Work out the finished part from the listing and answer in its coordinate system (mm). Face numbers are marked on the shaded views. A direction names the side the tool comes from. Coordinates: 2 decimals unless noted, no trailing zeros. Order: outer loops, then holes, each group sorted by start corner. A loop starts at its lowest first (then second) coordinate and runs counter-clockwise, first axis right, second up. Notation, with made-up numbers: (64.5, 21.5) - (70.5, 21.5) arc R28 ccw to (70.5, 58.5) - close; hole circle Ø4 at (50, -33). An arc over 180 degrees is marked (long way). Answer as a JSON object with one key per item and string values. Group by question number.
1) The mould has two halves that part along X. Classify the marked faces 1, 2 and 3: released by +X, released by -X, zero draft, split by the parting line, or undercut.
2) Each of these flat-tipped pins is pushed along its axis until it touches: P1, Ø10, axis at x = 10, y = 6.5, coming from the +Z side (3 decimals); P2, Ø3.5, axis at y = 19.05, z = 79.248, coming from the +X side; P3, Ø4, axis at x = -9, y = 8.5, coming from the -Z side; P4, Ø4.5, axis at y = 17.74, z = 10.92, coming from the -X side. Where does it stop, or does it pass through?
3) Section D-D (z = 9.5) is taken. Give the vertices of the cut face in (x, y).
4) Section C-C (x = -27.5) is taken. Give the vertices of the cut face in (y, z) (3 decimals), plus the area to 3 significant figures.
5) A tool of negligible diameter and unlimited length cuts with its end or side. For the marked faces 4 and 5, from which of +Z, -Z, +X, -X, +Y, -Y can it reach the whole face along a straight path? Write none if from no direction.
6) Section B-B (y = 23) is taken. Give the vertices of the cut face in (x, z) (3 decimals).
7) Find the intervals of material crossed by line 1 along X through (y, z) = (9.5, 63); line 2 along Y through (x, z) = (22.5, 16); line 3 along Y through (x, z) = (35.8, 52.07), in increasing order.
8) Section A-A (z = 52.07) is taken. Give the vertices of the cut face in (x, y), plus the area to 3 significant figures.
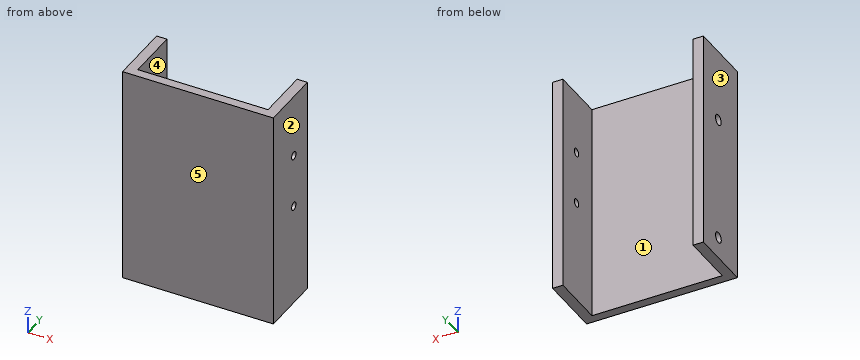
from build123d import *

# Parameters (mm, degrees)
BOSS_EXTRUDE3_DEPTH = 111.125
SKETCH4_R           = 2.667
CUT_EXTRUDE1_DEPTH  = 136.634929771
SKETCH5_R           = 2.667
CUT_EXTRUDE2_DEPTH  = 136.634929771
SKETCH6_R           = 2.032
CUT_EXTRUDE3_DEPTH  = 136.634929771
SKETCH7_R           = 2.032
CUT_EXTRUDE4_DEPTH  = 136.634929771


with BuildPart() as part:
    # Sketch2 → Boss-Extrude3 (new body)
    with BuildSketch(Plane.XY):
        Polygon((-38.1, 0), (38.1, 0), (38.1, 31.75), (32.893, 31.75), (32.893, 4.5974), (-32.893, 4.5974), (-32.893, 31.75), (-38.1, 31.75), align=None)
    extrude(amount=BOSS_EXTRUDE3_DEPTH)

    # Sketch4 → Cut-Extrude1 (cut, through all)
    with BuildSketch(Plane(origin=(-32.893, 0, 0), x_dir=(0, 0, -1), z_dir=(1, 0, 0))):
        with Locations((-10.922, 17.735211787)):
            Circle(SKETCH4_R)
    extrude(amount=-CUT_EXTRUDE1_DEPTH, mode=Mode.SUBTRACT)

    # Sketch5 → Cut-Extrude2 (cut, through all)
    with BuildSketch(Plane(origin=(-32.893, 0, 0), x_dir=(0, 0, -1), z_dir=(1, 0, 0))):
        with Locations((-74.295, 17.78)):
            Circle(SKETCH5_R)
    extrude(amount=-CUT_EXTRUDE2_DEPTH, mode=Mode.SUBTRACT)

    # Sketch6 → Cut-Extrude3 (cut, through all)
    with BuildSketch(Plane.ZY.offset(-32.893)):
        with Locations((52.07, 19.05)):
            Circle(SKETCH6_R)
    extrude(amount=-CUT_EXTRUDE3_DEPTH, mode=Mode.SUBTRACT)

    # Sketch7 → Cut-Extrude4 (cut, through all)
    with BuildSketch(Plane.ZY.offset(-32.893)):
        with Locations((79.248, 19.05)):
            Circle(SKETCH7_R)
    extrude(amount=-CUT_EXTRUDE4_DEPTH, mode=Mode.SUBTRACT)


solid = part.part
Report:
{
 "1": {"face 1": "undercut", "face 2": "released by +X", "face 3": "released by -X"},
 "2": {"P1": "stops at z = 111.125", "P2": "stops at x = -32.89", "P3": "passes through", "P4": "stops at x = 32.89"},
 "3": {"outline": "(-38.1, 0) - (38.1, 0) - (38.1, 31.75) - (32.89, 31.75) - (32.89, 4.6) - (-32.89, 4.6) - (-32.89, 15.48) - (-38.1, 15.48) - close; (-38.1, 19.99) - (-32.89, 19.99) - (-32.89, 31.75) - (-38.1, 31.75) - close"},
 "4": {"outline": "(0, 0) - (4.597, 0) - (4.597, 111.125) - (0, 111.125) - close", "area": "511 mm²"},
 "5": {"face 4": "+Z, -Z, +Y", "face 5": "+Z, -Z, +X, -X, -Y"},
 "6": {"outline": "(-38.1, 0) - (-32.893, 0) - (-32.893, 111.125) - (-38.1, 111.125) - close; (32.893, 0) - (38.1, 0) - (38.1, 111.125) - (32.893, 111.125) - close"},
 "7": {"line 1": "x = -38.1 to -32.89, 32.89 to 38.1", "line 2": "y = 0 to 4.6", "line 3": "y = 0 to 17.02, 21.08 to 31.75"},
 "8": {"outline": "(-38.1, 0) - (38.1, 0) - (38.1, 17.02) - (32.89, 17.02) - (32.89, 4.6) - (-32.89, 4.6) - (-32.89, 31.75) - (-38.1, 31.75) - close; (32.89, 21.08) - (38.1, 21.08) - (38.1, 31.75) - (32.89, 31.75) - close", "area": "612 mm²"}
}
